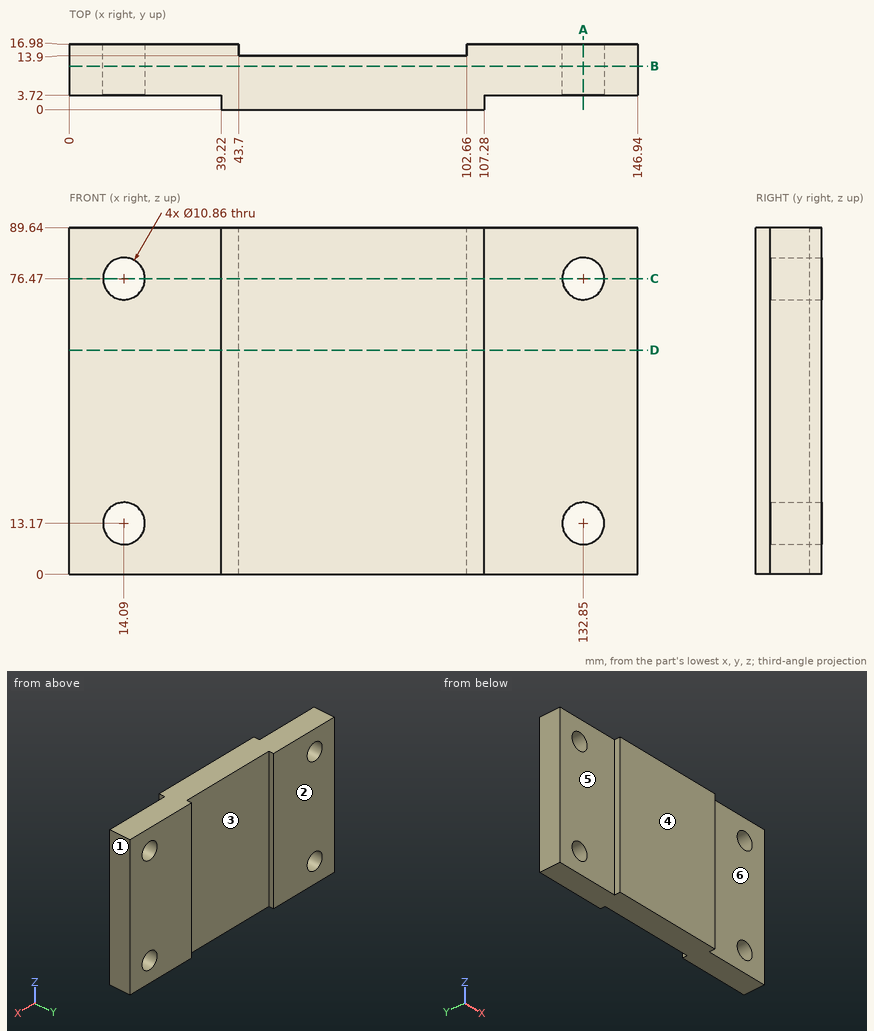
For this review, use the dimensioned drawing (mm, ordinates from the lowest corner) and the shaded views. A direction names the side the tool comes from. Give positions to 0.01 mm unless a question says otherwise; leave off trailing zeros. Loops run counter-clockwise (first coordinate to the right, second up) from the corner with the lowest first, then second, coordinate; pieces in that order, holes last.
Item 1: Take a section at B-B, the plane y = 11.25. State the section outline as (x, z) points.
Item 2: Take a section at C-C, the plane z = 76.47. State the section outline as (x, y) points, and give its area (3 significant figures).
Item 3: Tool access review of the marked faces 4, 5 and 6: name each direction out of +Z, -Z, +X, -X, +Y, -Y from which nothing blocks a thin tool from reaching the whole face with its end or side.
Item 4: Take a section at A-A, the plane x = 132.85. State the section outline as (y, z) points.
Item 5: Take a section at D-D, the plane z = 58. State the section outline as (x, y) points, and give its area (3 significant figures).
Item 6: Draft analysis for pull direction X (two halves, no side actions). For the marked faces 1, 2 and 3, state which applies: +X half, -X half, draft (parallel to the pull), parting line (faces both ways), or undercut.
Item 7: Insertion check: pin 1 (2 mm diameter, centred on x = 51, y = 11, fed in from -Z); pin 2 (10 mm diameter, centred on x = 132.85, z = 76.47, fed in from +Y); pin 3 (12.5 mm diameter, centred on x = 132.85, z = 13.17, fed in from -Y); pin 4 (3 mm diameter, centred on y = 2, z = 60, fed in from -X). Each pin has a flat end and moves straight along its axis. Give the tip position at first contact, or say it passes through.
Item 8: For line 1 along Z through (x, y) = (132.85, 7); line 2 along Z through (x, y) = (134, 16.25); line 3 along Y through (x, z) = (108, 44), list the stretches that pass through material, from the lowest coordinate up.
Calculated:
1. outline: (0, 0) - (146.94, 0) - (146.94, 89.64) - (0, 89.64) - close; hole circle Ø10.86 at (14.09, 13.17); hole circle Ø10.86 at (14.09, 76.47); hole circle Ø10.86 at (132.85, 13.17); hole circle Ø10.86 at (132.85, 76.47)
2. outline: (0, 3.72) - (8.66, 3.72) - (8.66, 16.98) - (0, 16.98) - close; (19.52, 3.72) - (39.22, 3.72) - (39.22, 0) - (107.28, 0) - (107.28, 3.72) - (127.42, 3.72) - (127.42, 16.98) - (102.66, 16.98) - (102.66, 13.9) - (43.7, 13.9) - (43.7, 16.98) - (19.52, 16.98) - close; (138.28, 3.72) - (146.94, 3.72) - (146.94, 16.98) - (138.28, 16.98) - close
2. area: 1,730 mm2
3. face 4: +Z, -Z, +X, -X, -Y
3. face 5: +Z, -Z, -X, -Y
3. face 6: +Z, -Z, +X, -Y
4. outline: (3.72, 0) - (16.98, 0) - (16.98, 7.74) - (3.72, 7.74) - close; (3.72, 18.6) - (16.98, 18.6) - (16.98, 71.04) - (3.72, 71.04) - close; (3.72, 81.9) - (16.98, 81.9) - (16.98, 89.64) - (3.72, 89.64) - close
5. outline: (0, 3.72) - (39.22, 3.72) - (39.22, 0) - (107.28, 0) - (107.28, 3.72) - (146.94, 3.72) - (146.94, 16.98) - (102.66, 16.98) - (102.66, 13.9) - (43.7, 13.9) - (43.7, 16.98) - (0, 16.98) - close
5. area: 2,020 mm2
6. face 1: +X half
6. face 2: draft
6. face 3: undercut
7. pin 1: stops at z = 0
7. pin 2: passes through
7. pin 3: stops at y = 3.72
7. pin 4: stops at x = 39.22
8. line 1: z = 0 to 7.74, 18.6 to 71.04, 81.9 to 89.64
8. line 2: z = 0 to 7.86, 18.48 to 71.16, 81.78 to 89.64
8. line 3: y = 3.72 to 16.98
